from build123d import *

# Parameters (mm, degrees)
BOSS_EXTRUDE1_DEPTH     = 85
SKETCH3_R               = 5
BOSS_EXTRUDE2_DEPTH     = 57.5
BOSS_EXTRUDE3_START     = -25
BOSS_EXTRUDE3_DEPTH     = 56.666666667
BOSS_EXTRUDE4_DEPTH     = 2.5
FILLET2_R               = 10
CUT_EXTRUDE1_DEPTH      = 86
CUT_EXTRUDE1_DEPTH_BACK = 26


with BuildPart() as part:
    # Sketch2 → Boss-Extrude1 (new body)
    with BuildSketch(Plane(origin=(0, 0, 0), x_dir=(1, 0, 0), z_dir=(0, 1, 0))):
        Polygon((0, -57.5), (0, 57.5), (-85, 0), align=None)
        Polygon((-10, 38.662131911), (-67.152716738, 0), (-10, -38.662131911), align=None, mode=Mode.SUBTRACT)
    extrude(amount=BOSS_EXTRUDE1_DEPTH)

    # Sketch3 → Boss-Extrude2 (add, symmetric)
    with BuildSketch(Plane.XY):
        with BuildLine():
            Line((0, 0), (50, 0))
            Line((50, 0), (91.711375741, 35))
            Line((91.711375741, 35), (134.654022129, 35))
            Line((134.654022129, 35), (185, -25))
            Line((185, -25), (230, -25))
            Line((230, -25), (230, -19))
            Line((230, -19), (230, -5))
            Line((230, -5), (215, -5))
            ThreePointArc((215, -5), (207.928932188, -7.928932188), (205, -15))
            Line((205, -15), (205, -19))
            Line((205, -19), (187.797845949, -19))
            Line((187.797845949, -19), (137.451868078, 41))
            Line((137.451868078, 41), (89.527554335, 41))
            Line((89.527554335, 41), (47.816178594, 6))
            Line((47.816178594, 6), (33.75, 6))
            Line((33.75, 6), (33.75, 10))
            ThreePointArc((33.75, 10), (30.821067812, 17.071067812), (23.75, 20))
            Line((23.75, 20), (0, 20))
            Line((0, 20), (0, 0))
        make_face()
        with Locations((23.75, 10)):
            Circle(SKETCH3_R, mode=Mode.SUBTRACT)
        with Locations((215, -15)):
            Circle(SKETCH3_R, mode=Mode.SUBTRACT)
    extrude(amount=BOSS_EXTRUDE2_DEPTH, both=True)

    # Sketch4 → Boss-Extrude3 (add)
    with BuildSketch(Plane(origin=(0, 0, 0), x_dir=(1, 0, 0), z_dir=(0, 1, 0)).offset(BOSS_EXTRUDE3_START)):
        Polygon((230, -30), (230, 30), (275, 0), align=None)
        Polygon((240, 11.314829082), (256.972243623, 0), (240, -11.314829082), align=None, mode=Mode.SUBTRACT)
    extrude(amount=BOSS_EXTRUDE3_DEPTH)

    # Sketch5 → Boss-Extrude4 (add, symmetric)
    with BuildSketch(Plane.XY):
        with BuildLine():
            Line((0, 85), (166.672120299, 85))
            Line((166.672120299, 85), (211.424100629, 31.666666667))
            Line((211.424100629, 31.666666667), (230, 31.666666667))
            Line((230, 31.666666667), (230, -5))
            Line((230, -5), (215, -5))
            ThreePointArc((215, -5), (207.928932188, -7.928932188), (205, -15))
            Line((205, -15), (205, -19))
            Line((205, -19), (187.797845949, -19))
            Line((187.797845949, -19), (137.451868078, 41))
            Line((137.451868078, 41), (89.527554335, 41))
            Line((89.527554335, 41), (47.816178594, 6))
            Line((47.816178594, 6), (33.75, 6))
            Line((33.75, 6), (33.75, 10))
            ThreePointArc((33.75, 10), (30.821067812, 17.071067812), (23.75, 20))
            Line((23.75, 20), (0, 20))
            Line((0, 20), (0, 85))
        make_face()
    extrude(amount=BOSS_EXTRUDE4_DEPTH, both=True)

    # Fillet2
    fillet2_edges = [part.edges().sort_by_distance(p)[0] for p in [
        (211.424100629, 31.666666667, 0),
        (166.672120299, 85, 0),
        (50, 0, 0),
        (91.711375741, 35, 0),
        (134.654022129, 35, 0),
        (185, -25, 0),
        (187.797845949, -19, 30),
        (137.451868078, 41, 30),
        (89.527554335, 41, 30),
        (47.816178594, 6, 30),
        (47.816178594, 6, -30),
        (89.527554335, 41, -30),
        (137.451868078, 41, -30),
        (187.797845949, -19, -30),
    ]]
    fillet(fillet2_edges, radius=FILLET2_R)

    # Sketch6 → Cut-Extrude1 (cut, two sides)
    with BuildSketch(Plane(origin=(0, 0, 0), x_dir=(1, 0, 0), z_dir=(0, 1, 0))) as cut_extrude1_sk:
        Polygon((0, 57.5), (230, 57.5), (230, 30), align=None)
        Polygon((0, -57.5), (230, -30), (230, -57.5), align=None)
    extrude(amount=CUT_EXTRUDE1_DEPTH, mode=Mode.SUBTRACT)
    extrude(cut_extrude1_sk.sketch, amount=-CUT_EXTRUDE1_DEPTH_BACK, mode=Mode.SUBTRACT)


solid = part.part
Work out the finished part from the listing and answer in its coordinate system (mm). A direction names the side the tool comes from. Round coordinates to 2 decimals unless told otherwise and drop trailing zeros. Write each loop counter-clockwise with the first axis right and the second up, starting at its lowest first coordinate (ties: lowest second). Pieces come first, ordered by that corner, then holes.
1) A cutting plane is placed at B-B (x = -59). Give the vertices of the cut face in (y, z).
2) A tool of negligible diameter and unlimited length cuts with its end or side. For faces 5 (the flat face through (-38.98, 41.9, 19.06)), 6 (the flat face through (239, 31.667, 0)), 7 (the cylindrical face through (49.735, 0.586, 0.727)), 8 (the flat face through (39, 6, -28)), from which of +Z, -Z, +X, -X, +Y, -Y can it reach the whole face along a straight path? Write none if from no direction.
3) Given pin 1 Ø11.5 at (x, z) = (40.5, -23.5) entering from +Y; pin 2 Ø2 at (y, z) = (9, -8) entering from -X; pin 3 Ø3 at (y, z) = (8, 24) entering from +X, each flat-ended and moving along its own axis, determine where each tip first touches the part or whether it passes through.
4) The mould has two halves that part along X. Classify faces 1 (the flat face through (39, 6, 28)), 2 (the flat face through (9, 0, 1)), 3 (the flat face through (252.2, 2.9, -15.2)), 4 (the flat face through (-10, 42, 1)): pulls with the +X half, pulls with the -X half, needs draft (parallel to the pull), parting line crosses it, or undercut.
5) A cutting plane is placed at A-A (y = 24). Give the vertices of the cut face in (x, z).
6) Straight lines are drawn through the part: line 1 (Y direction, x = 215, z = -11); line 2 (X direction, y = 10, z = -23.5); line 3 (Y direction, x = 23.75, z = 20.5). For each, find the intervals that lie inside material, in ascending order.
Completed:
1. outline: (0, -17.59) - (85, -17.59) - (85, -5.52) - (0, -5.52) - close; (0, 5.52) - (85, 5.52) - (85, 17.59) - (0, 17.59) - close
2. face 5: +Y, -Y
2. face 6: +Z, -Z, +X, +Y
2. face 7: +Z, -Z, -Y
2. face 8: -Z, +Y
3. pin 1: stops at y = 6.22
3. pin 2: stops at x = -74.65
3. pin 3: stops at x = 241.25
4. face 1: undercut
4. face 2: needs draft
4. face 3: pulls with the +X half
4. face 4: undercut
5. outline: (-85, 0) - (0, -57.5) - (0, -2.5) - (69.27, -2.5) - (69.27, -49.22) - (78.6, -48.1) - (78.6, 48.1) - (69.27, 49.22) - (69.27, 2.5) - (0, 2.5) - (0, 57.5) - close; (143.88, -40.3) - (151.72, -39.36) - (151.72, -2.5) - (230, -2.5) - (230, -30) - (275, 0) - (230, 30) - (230, 2.5) - (151.72, 2.5) - (151.72, 39.36) - (143.88, 40.3) - close; hole (-67.15, 0) - (-10, -38.66) - (-10, 38.66) - close; hole (240, -11.31) - (256.97, 0) - (240, 11.31) - close
6. line 1: y = -25 to -20, -10 to -5
6. line 2: x = -50.26 to -32.41, -10 to 18.75, 28.75 to 33.75, 52.58 to 61.92, 155.63 to 163.46, 230 to 239.75
6. line 3: y = 0 to 5, 15 to 20
